from build123d import *

# Parameters (mm, degrees)
SKETCH3_R           = 45.8838883
CUT_EXTRUDE1_DEPTH  = 16
BOSS_EXTRUDE1_DEPTH = 31
CIRPATTERN1_COUNT   = 8


with BuildPart() as part:
    # Sketch1 → Revolve1 (revolve)
    with BuildSketch(Plane.XY):
        Polygon((0, -25), (23.5, -25), (23.5, -20.15), (47, -20.15), (47, -24.15), (67, -24.15), (67, -28), (51, -28), (51, -39.5), (20, -39.5), (20, -34), (0, -34), align=None)
    revolve(axis=Axis((0, 0, 0), (1, 0, 0)))

    # Sketch3 → Cut-Extrude1 (cut)
    with BuildSketch(Plane(origin=(67, 0, 0), x_dir=(0, 0, -1), z_dir=(1, 0, 0))):
        Circle(SKETCH3_R)
        Polygon((0, 29.224589408), (-20.664905348, 20.664905348), (-29.224589408, 0), (-20.664905348, -20.664905348), (0, -29.224589408), (20.664905348, -20.664905348), (29.224589408, 0), (20.664905348, 20.664905348), align=None, mode=Mode.SUBTRACT)
    extrude(amount=-CUT_EXTRUDE1_DEPTH, mode=Mode.SUBTRACT)

    # Sketch4 → Boss-Extrude1 (add)
    with BuildSketch(Plane(origin=(51, 0, 0), x_dir=(0, 0, -1), z_dir=(1, 0, 0))):
        with BuildLine():
            Line((-3.822673778, 39.492546862), (-5, 39.182266397))
            Line((-5, 39.182266397), (5, 39.182266397))
            Line((5, 39.182266397), (3.822673778, 39.492546862))
            ThreePointArc((3.822673778, 39.492546862), (0, 39.987817799), (-3.822673778, 39.492546862))
        make_face()
    boss_extrude1 = extrude(amount=-BOSS_EXTRUDE1_DEPTH)

    # CirPattern1: Boss-Extrude1 ×8 about axis
    cirpattern1_axis = Axis((0, 0, 0), (1, 0, 0))
    for i in range(1, CIRPATTERN1_COUNT):
        add(boss_extrude1.rotate(cirpattern1_axis, i * 360 / CIRPATTERN1_COUNT))


solid = part.part
The listing builds one solid part. Answer for the finished solid, in the listing's coordinates (mm). A direction names the side the tool comes from. Coordinates: 2 decimals unless noted, no trailing zeros. Loops run counter-clockwise (first coordinate to the right, second up) from the corner with the lowest first, then second, coordinate; pieces in that order, holes last.
1) Find section A-A on y = 0. Write down the section's boundary in (x, z).
2) Find section D-D on x = 8. Write down the section's boundary in (y, z).
3) Flat-ended cylindrical pins translate along their axes: pin 1 Ø8 at (x, y) = (56, 9.5) entering from -Z; pin 2 Ø5 at (x, z) = (22.5, 19.5) entering from -Y; pin 3 Ø4 at (y, z) = (-26.5, 20) entering from +X; pin 4 Ø14.5 at (y, z) = (7, -7.5) entering from +X. Find the tip coordinate at first contact, or state that the pin passes through.
4) Find the intervals of material crossed by L1, parallel to Z at x = 5.5, y = 0; L2, parallel to Z at x = 59, y = 0, in increasing order.
5) A tool of negligible diameter and unlimited length cuts with its end or side. For faces 1 (the face through (59.112, 10.428, 24.905)), 2 (the face through (59.112, -24.905, 10.428)), 3 (the face through (9.86, -18.28, -28.67)), 4 (the face through (59.1, 10.2, -25)), 5 (the face through (57.14, 24.127, -1.062)), from which of +Z, -Z, +X, -X, +Y, -Y can it reach the whole face along a straight path? Write none if from no direction.
Values:
1. outline: (0, -34) - (20, -34) - (20, -39.99) - (51, -39.99) - (51, -28) - (67, -28) - (67, -24.15) - (47, -24.15) - (47, -20.15) - (23.5, -20.15) - (23.5, -25) - (0, -25) - close; (0, 25) - (23.5, 25) - (23.5, 20.15) - (47, 20.15) - (47, 24.15) - (67, 24.15) - (67, 28) - (51, 28) - (51, 39.99) - (20, 39.99) - (20, 34) - (0, 34) - close
2. outline: circle Ø68 at (0, 0); hole circle Ø50 at (0, 0)
3. pin 1: stops at z = -26.95
3. pin 2: stops at y = -35.65
3. pin 3: stops at x = 51
3. pin 4: passes through
4. L1: z = -34 to -25, 25 to 34
4. L2: z = -28 to -24.15, 24.15 to 28
5. face 1: +Z, +X, +Y
5. face 2: +Z, +X, -Y
5. face 3: -X
5. face 4: -Z, +X, +Y
5. face 5: +X
